from build123d import *

# Parameters (mm, degrees)
F0_R     = 8.75
F3_DEPTH = 3
F1_R     = 7
F4_DEPTH = 9
F5_DEPTH = 15
F6_W     = 3
F6_H     = 9
F7_DEPTH = 20
F8_SIZE  = 0.5


with BuildPart() as f3:
    # F0 (on Top) → F3 (new body)
    with BuildSketch(Plane.XY):
        Circle(F0_R)
    extrude(amount=F3_DEPTH)

    # F1 (on Top) → F4 (join)
    with BuildSketch(Plane.XY):
        Circle(F1_R)
    extrude(amount=-F4_DEPTH)

    # F2 (on Top) → F5 (join)
    with BuildSketch(Plane.XY):
        with BuildLine():
            Line((4.5, -3.1622776602), (4.5, 3.1622776602))
            ThreePointArc((4.5, 3.1622776602), (0, 5.5), (-4.5, 3.1622776602))
            Line((-4.5, 3.1622776602), (-4.5, -3.1622776602))
            ThreePointArc((-4.5, -3.1622776602), (0, -5.5), (4.5, -3.1622776602))
        make_face()
    extrude(amount=-F5_DEPTH)

    # F6 (on Top) → F7 (cut, symmetric)
    with BuildSketch(Plane.XY):
        Rectangle(F6_W, F6_H)
    extrude(amount=F7_DEPTH, both=True, mode=Mode.SUBTRACT)

    # F8
    f8_edges = [f3.edges().sort_by_distance(p)[0] for p in [
        (-8.75, 0, 3),
        (-1.5, 0, 3),
        (0, -4.5, 3),
        (1.5, 0, 3),
        (0, 4.5, 3),
    ]]
    chamfer(f8_edges, length=F8_SIZE)


solid = f3.part
Input: part model. Units: mm. Frame: model coordinates. A direction names the side the tool comes from. Coordinates: 2 decimals unless noted, no trailing zeros. Order: outer loops, then holes, each group sorted by start corner. A loop starts at its lowest first (then second) coordinate and runs counter-clockwise, first axis right, second up.
1. Cut plane A-A, the plane y = 0. Return loops of the section in (x, z), plus the area to 3 significant figures.
Checked values:
outline: (-8.75, 0) - (-7, 0) - (-7, -9) - (-4.5, -9) - (-4.5, -15) - (-1.5, -15) - (-1.5, 2.5) - (-2, 3) - (-8.25, 3) - (-8.75, 2.5) - close; (1.5, -15) - (4.5, -15) - (4.5, -9) - (7, -9) - (7, 0) - (8.75, 0) - (8.75, 2.5) - (8.25, 3) - (2, 3) - (1.5, 2.5) - close
area: 178 mm2
2. Cut plane C-C, the plane z = -1.25. Return loops of the section in (x, y).
Checked values:
outline: circle Ø14 at (0, 0); hole (-1.5, -4.5) - (1.5, -4.5) - (1.5, 4.5) - (-1.5, 4.5) - close
3. Draft query along X for faces 1 (the flat face through (0, -4.5, -6)), 2 (the flat face through (-4, 6, 0)), 3 (the flat face through (4.5, 0, -12)), 4 (the flat face through (-4.5, 0, -12)). Return one class per face: +X half, -X half, draft (parallel to the pull), parting line (faces both ways), or undercut.
Checked values:
face 1: undercut
face 2: draft
face 3: +X half
face 4: -X half
4. Contact query for flat-ended pins moving along their axis: P1, Ø6, axis at x = 2, z = -5, coming from the +Y side; P2, Ø5, axis at y = -1.5, z = -12, coming from the +X side; P3, Ø5, axis at x = 3.5, y = 6.5, coming from the -Z side; P4, Ø6.5, axis at y = 0.5, z = -13, coming from the -X side. Output: stop coordinate, or through.
Checked values:
P1: stops at y = 7
P2: stops at x = 4.5
P3: stops at z = -15
P4: stops at x = -4.5
5. Cut plane B-B, the plane x = 0. Return loops of the section in (y, z).
Checked values:
outline: (-8.75, 0) - (-7, 0) - (-7, -9) - (-5.5, -9) - (-5.5, -15) - (-4.5, -15) - (-4.5, 2.5) - (-5, 3) - (-8.25, 3) - (-8.75, 2.5) - close; (4.5, -15) - (5.5, -15) - (5.5, -9) - (7, -9) - (7, 0) - (8.75, 0) - (8.75, 2.5) - (8.25, 3) - (5, 3) - (4.5, 2.5) - close
6. Access query for faces 5 (the cylindrical face through (0.1, 5.5, -12)), 6 (the cylindrical face through (6.466, -2.681, -4.437)), 7 (the flat face through (4, 0, 3)), 8 (the flat face through (-1.5, 0, -6)), 9 (the cylindrical face through (-0.1, -5.5, -12)). Directions: +Z, -Z, +X, -X, +Y, -Y. A direction counts if a zero-diameter tool reaches every point of the face in a straight line with its end or side. Return the directions, or none.
Checked values:
face 5: -Z, +Y
face 6: -Z
face 7: +Z, +X, -X, +Y, -Y
face 8: +Z, -Z
face 9: -Z, -Y
7. Ray query, line 1 along X through (y, z) = (1, -9.25); line 2 along Z through (x, y) = (-5.5, -2); line 3 along Y through (x, z) = (0.75, -5.5). Return the intervals inside material, ascending.
Checked values:
line 1: x = -4.5 to -1.5, 1.5 to 4.5
line 2: z = -9 to 3
line 3: y = -6.96 to -4.5, 4.5 to 6.96
